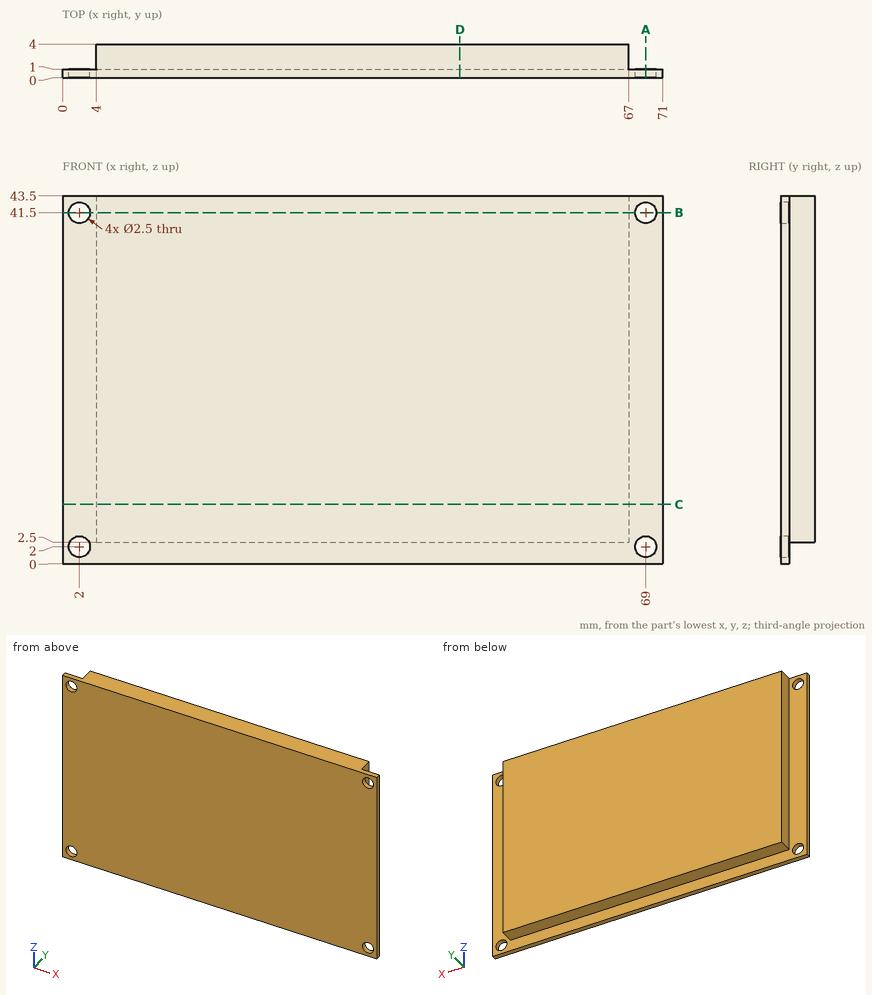
Study the drawing (mm; zero at the part's minimum x, y, z) and answer. Coordinates: 2 decimals unless noted, no trailing zeros. Loops run counter-clockwise (first coordinate to the right, second up) from the corner with the lowest first, then second, coordinate; pieces in that order, holes last. Notation, with made-up numbers: M -31,14.5 L -15,14.5 A25 cw -15,50.5 Z; hole C 55.25,-1 d10. An arc over 180 degrees is marked long. Answer in a Markdown table with one row per item.
1) Find section B-B (z = 41.5). Determine the outline of the cut face in (x, y).
Answers below:
| item | result |
|---|---|
| outline | M 0,0 L 0.75,0 L 0.75,1 L 0,1 Z; M 3.25,0 L 67.75,0 L 67.75,1 L 67,1 L 67,4 L 4,4 L 4,1 L 3.25,1 Z; M 70.25,0 L 71,0 L 71,1 L 70.25,1 Z |
2) Given pin 1 (1.5 mm diameter, centred on y = 3, z = 16, fed in from +X); pin 2 (2 mm diameter, centred on x = 69, z = 41.5, fed in from -Y); pin 3 (1.5 mm diameter, centred on y = 2, z = 13, fed in from -X); pin 4 (3 mm diameter, centred on x = 69, z = 2, fed in from +Y), each flat-ended and moving along its own axis, determine where each tip first touches the part or whether it passes through.
Answers below:
| item | result |
|---|---|
| pin 1 | x = 67 |
| pin 2 | through |
| pin 3 | x = 4 |
| pin 4 | y = 1 |
3) Find section A-A (x = 69). Determine the outline of the cut face in (y, z).
Answers below:
| item | result |
|---|---|
| outline | M 0,0 L 1,0 L 1,0.75 L 0,0.75 Z; M 0,3.25 L 1,3.25 L 1,40.25 L 0,40.25 Z; M 0,42.75 L 1,42.75 L 1,43.5 L 0,43.5 Z |
4) Find section C-C (z = 7). Determine the outline of the cut face in (x, y), then the cut area to 3 significant figures.
Answers below:
| item | result |
|---|---|
| outline | M 0,0 L 71,0 L 71,1 L 67,1 L 67,4 L 4,4 L 4,1 L 0,1 Z |
| area | 260 mm^2 |
5) Find the intervals of material crossed by probe 1 along X at (y, z) = (0.55, 2); probe 2 along X at (y, z) = (3.3, 15.5); probe 3 along Z at (x, y) = (66, 2.05), in increasing order.
Answers below:
| item | result |
|---|---|
| probe 1 | 0 to 0.75, 3.25 to 67.75, 70.25 to 71 |
| probe 2 | 4 to 67 |
| probe 3 | 2.5 to 43.5 |
6) Find section D-D (x = 47). Determine the outline of the cut face in (y, z).
Answers below:
| item | result |
|---|---|
| outline | M 0,0 L 1,0 L 1,2.5 L 4,2.5 L 4,43.5 L 0,43.5 Z |
